```python
from build123d import *

# Parameters (mm, degrees)
BASE_SKETCH_W                   = 16
BASE_SKETCH_H                   = 20
BASE_EXTRUDE_DEPTH              = 12
TOP_START                       = 10
PROTRUSION_SKETCH_R             = 5
TOP_PROTRUSION_EXTRUDE_DEPTH    = 2
BOTTOM_START                    = -10
PROTRUSION_SKETCH_2_R           = 5
BOTTOM_PROTRUSION_EXTRUDE_DEPTH = 2
PROTRUSION_CHAMFER_SIZE         = 1
F_5_0MM_DOWEL_HOLE1_D           = 5
F_1_6MM_DOWEL_HOLE1_D           = 1.6
F_1_6MM_DOWEL_HOLE1_DEPTH       = 8
F_1_6MM_DOWEL_HOLE1_TIP         = 0.480688495
F_1_6_1_6_DIAMETER_HOLE4_D      = 1.6
F_1_6_1_6_DIAMETER_HOLE4_DEPTH  = 3.5
F_1_6_1_6_DIAMETER_HOLE4_TIP    = 0.480688495
M2X0_4_TAPPED_HOLE1_D           = 1.6
M2X0_4_TAPPED_HOLE1_DEPTH       = 4
M2X0_4_TAPPED_HOLE1_TIP         = 0.480688495
M2X0_4_TAPPED_HOLE2_D           = 1.6
M2X0_4_TAPPED_HOLE2_DEPTH       = 4
M2X0_4_TAPPED_HOLE2_TIP         = 0.480688495
F_2_2_2_2_DIAMETER_HOLE1_D      = 2.2
F_1_3_1_3_DIAMETER_HOLE1_D      = 1.3
F_1_3_1_3_DIAMETER_HOLE1_DEPTH  = 6
F_1_3_1_3_DIAMETER_HOLE1_TIP    = 0.390559402
F_1_3_1_3_DIAMETER_HOLE2_D      = 1.3
F_1_3_1_3_DIAMETER_HOLE2_DEPTH  = 6
F_1_3_1_3_DIAMETER_HOLE2_TIP    = 0.390559402
F_1_3_1_3_DIAMETER_HOLE3_D      = 1.3
F_1_3_1_3_DIAMETER_HOLE3_DEPTH  = 6
F_1_3_1_3_DIAMETER_HOLE3_TIP    = 0.390559402


with BuildPart() as part:
    # Base Sketch → Base Extrude (new body)
    with BuildSketch(Plane(origin=(0, 0, 0), x_dir=(1, 0, 0), z_dir=(0, 1, 0))):
        Rectangle(BASE_SKETCH_W, BASE_SKETCH_H)
    extrude(amount=BASE_EXTRUDE_DEPTH)

    # Protrusion Sketch → Top Protrusion Extrude (add)
    with BuildSketch(Plane.XY.offset(TOP_START)):
        with Locations((0, 6)):
            Circle(PROTRUSION_SKETCH_R)
    extrude(amount=TOP_PROTRUSION_EXTRUDE_DEPTH)

    # Protrusion Sketch<2> → Bottom Protrusion Extrude (add)
    with BuildSketch(Plane.XY.offset(BOTTOM_START)):
        with Locations((0, 6)):
            Circle(PROTRUSION_SKETCH_2_R)
    extrude(amount=-BOTTOM_PROTRUSION_EXTRUDE_DEPTH)

    # Protrusion Chamfer
    protrusion_chamfer_edges = [part.edges().sort_by_distance(p)[0] for p in [
        (-5, 6, 12),
        (-5, 6, -12),
    ]]
    chamfer(protrusion_chamfer_edges, length=PROTRUSION_CHAMFER_SIZE)

    # Ø5.0mm Dowel Hole1 (through all)
    with Locations(Plane.XY.offset(12)):
        with Locations((0, 6)):
            Hole(F_5_0MM_DOWEL_HOLE1_D / 2)

    # Ø1.6mm Dowel Hole1
    with Locations(Plane(origin=(8, 0, 0), x_dir=(0, 0, -1), z_dir=(1, 0, 0))):
        with Locations((0, 6)):
            Hole(F_1_6MM_DOWEL_HOLE1_D / 2, depth=F_1_6MM_DOWEL_HOLE1_DEPTH)
            with Locations((0, 0, -(F_1_6MM_DOWEL_HOLE1_DEPTH + F_1_6MM_DOWEL_HOLE1_TIP / 2))):  # 118° drill point
                Cone(0, F_1_6MM_DOWEL_HOLE1_D / 2, F_1_6MM_DOWEL_HOLE1_TIP, mode=Mode.SUBTRACT)

    # Ø1.6 (1.6) Diameter Hole4
    with Locations(Plane.ZY.offset(8)):
        with Locations((0, 6)):
            Hole(F_1_6_1_6_DIAMETER_HOLE4_D / 2, depth=F_1_6_1_6_DIAMETER_HOLE4_DEPTH)
            with Locations((0, 0, -(F_1_6_1_6_DIAMETER_HOLE4_DEPTH + F_1_6_1_6_DIAMETER_HOLE4_TIP / 2))):  # 118° drill point
                Cone(0, F_1_6_1_6_DIAMETER_HOLE4_D / 2, F_1_6_1_6_DIAMETER_HOLE4_TIP, mode=Mode.SUBTRACT)

    # M2x0.4 Tapped Hole1
    with Locations(Plane(origin=(8, 0, 0), x_dir=(0, 0, -1), z_dir=(1, 0, 0))):
        with Locations((-4.5, 6), (4.5, 6)):
            Hole(M2X0_4_TAPPED_HOLE1_D / 2, depth=M2X0_4_TAPPED_HOLE1_DEPTH)
            with Locations((0, 0, -(M2X0_4_TAPPED_HOLE1_DEPTH + M2X0_4_TAPPED_HOLE1_TIP / 2))):  # 118° drill point
                Cone(0, M2X0_4_TAPPED_HOLE1_D / 2, M2X0_4_TAPPED_HOLE1_TIP, mode=Mode.SUBTRACT)

    # M2x0.4 Tapped Hole2
    with Locations(Plane.ZY.offset(8)):
        with Locations((-4.5, 6), (4.5, 6)):
            Hole(M2X0_4_TAPPED_HOLE2_D / 2, depth=M2X0_4_TAPPED_HOLE2_DEPTH)
            with Locations((0, 0, -(M2X0_4_TAPPED_HOLE2_DEPTH + M2X0_4_TAPPED_HOLE2_TIP / 2))):  # 118° drill point
                Cone(0, M2X0_4_TAPPED_HOLE2_D / 2, M2X0_4_TAPPED_HOLE2_TIP, mode=Mode.SUBTRACT)

    # Ø2.2 (2.2) Diameter Hole1 (through all)
    with Locations(Plane(origin=(0, 12, 0), x_dir=(1, 0, 0), z_dir=(0, 1, 0))):
        with Locations((-5, 7), (5, 7), (-5, -7), (5, -7)):
            Hole(F_2_2_2_2_DIAMETER_HOLE1_D / 2)

    # Ø1.3 (1.3) Diameter Hole1
    with Locations(Plane(origin=(0, 0, 0), x_dir=(-1, 0, 0), z_dir=(0, -1, 0))):
        with Locations((0, 7.5), (0, -7.5)):
            Hole(F_1_3_1_3_DIAMETER_HOLE1_D / 2, depth=F_1_3_1_3_DIAMETER_HOLE1_DEPTH)
            with Locations((0, 0, -(F_1_3_1_3_DIAMETER_HOLE1_DEPTH + F_1_3_1_3_DIAMETER_HOLE1_TIP / 2))):  # 118° drill point
                Cone(0, F_1_3_1_3_DIAMETER_HOLE1_D / 2, F_1_3_1_3_DIAMETER_HOLE1_TIP, mode=Mode.SUBTRACT)

    # Ø1.3 (1.3) Diameter Hole2
    with Locations(Plane(origin=(0, 0, 0), x_dir=(-1, 0, 0), z_dir=(0, -1, 0))):
        with Locations((5, 0)):
            Hole(F_1_3_1_3_DIAMETER_HOLE2_D / 2, depth=F_1_3_1_3_DIAMETER_HOLE2_DEPTH)
            with Locations((0, 0, -(F_1_3_1_3_DIAMETER_HOLE2_DEPTH + F_1_3_1_3_DIAMETER_HOLE2_TIP / 2))):  # 118° drill point
                Cone(0, F_1_3_1_3_DIAMETER_HOLE2_D / 2, F_1_3_1_3_DIAMETER_HOLE2_TIP, mode=Mode.SUBTRACT)

    # Ø1.3 (1.3) Diameter Hole3
    with Locations(Plane(origin=(0, 12, 0), x_dir=(1, 0, 0), z_dir=(0, 1, 0))):
        with Locations((0, -7.5), (0, -3), (0, 3), (0, 7.5)):
            Hole(F_1_3_1_3_DIAMETER_HOLE3_D / 2, depth=F_1_3_1_3_DIAMETER_HOLE3_DEPTH)
            with Locations((0, 0, -(F_1_3_1_3_DIAMETER_HOLE3_DEPTH + F_1_3_1_3_DIAMETER_HOLE3_TIP / 2))):  # 118° drill point
                Cone(0, F_1_3_1_3_DIAMETER_HOLE3_D / 2, F_1_3_1_3_DIAMETER_HOLE3_TIP, mode=Mode.SUBTRACT)


solid = part.part
```
Part model, mm, in its own coordinate system. A direction names the side the tool comes from. Round coordinates to 2 decimals unless told otherwise and drop trailing zeros. Order: outer loops, then holes, each group sorted by start corner. A loop starts at its lowest first (then second) coordinate and runs counter-clockwise, first axis right, second up. Notation, with made-up numbers: M 18.25,-30 L 23.25,-30 A28 ccw 23.25,-6 Z; hole C 41.5,65 d5. An arc over 180 degrees is marked long. Answer in a Markdown table with one row per item. Add a question column.
Q1. Cut at C-C on z = 9.25. Give the cut face in (x, y).
Q2. Wall check: L1, parallel to Z at x = 0, y = 2.25; L2, parallel to Z at x = 5, y = 2.75; L3, parallel to Z at x = 0, y = 9.3. Give the ranges that are in metal, low to high. Write a range as from..to.
Q3. Pin check, flat tips, straight feed: pin 1 (1 mm diameter, centred on x = 0, z = -3, fed in from +Y); pin 2 (1 mm diameter, centred on x = 0, z = -7.5, fed in from +Y); pin 3 (2.5 mm diameter, centred on y = 6, z = -4.5, fed in from +X); pin 4 (1.3 mm diameter, centred on y = 6, z = 4.5, fed in from +X). Stop position of each tip, or through.
Q4. Cut at A-A on x = 6.5. Give the cut face in (y, z).
Q5. Cut at D-D on x = 0. Give the number of separate pieces and of enclosed holes in the cut face, and give its area (3 significant figures).
Q6. 3-axis set-ups, long thin cutter, end or side, ignore diameter. For faces 4 (the face through (-5.97, 6.54, -3.91)), 5 (the face through (-1.08, 1.12, 10.49)), 6 (the face through (-4.38, 2.81, -0.2)), 7 (the face through (5.97, 6.54, -5.09)): which of +Z, -Z, +X, -X, +Y, -Y reach the whole face in a straight line?
Q7. Mould opens along X. For faces 1 (the face through (-5.4, 5.9, 10)), 2 (the face through (-4.103, 6.138, -0.018)), 3 (the face through (0.35, 1.82, -8.05)) say: +X half, -X half, draft (parallel to the pull), parting line (faces both ways), or undercut.
Q8. Cut at B-B on z = -3. Give the cut face in (x, y).
Established:
| question | item | result |
|---|---|---|
| 1 | outline | M -8,0 L 8,0 L 8,12 L -8,12 Z; hole C 0,6 d5 |
| 2 | L1 | z = -12..-8.15, -6.85..6.85, 8.15..12 |
| 2 | L2 | z = -10..-8.1, -5.9..5.9, 8.1..10 |
| 2 | L3 | z = -12..-8.15, -6.85..-3.65, -2.35..2.35, 3.65..6.85, 8.15..12 |
| 3 | pin 1 | stops at y = 3.55 |
| 3 | pin 2 | passes through |
| 3 | pin 3 | stops at x = 8 |
| 3 | pin 4 | stops at x = 3.91 |
| 4 | outline | M 0,-10 L 12,-10 L 12,10 L 0,10 Z; hole C 6,-4.5 d1.6; hole C 6,0 d1.6; hole C 6,4.5 d1.6 |
| 5 | separate pieces | 8 |
| 5 | enclosed holes | 0 |
| 5 | area | 131 mm2 |
| 6 | face 4 | -X |
| 6 | face 5 | +Z |
| 6 | face 6 | -Y |
| 6 | face 7 | +X |
| 7 | face 1 | draft |
| 7 | face 2 | -X half |
| 7 | face 3 | undercut |
| 8 | outline | M -8,0 L 8,0 L 8,12 L 0.65,12 L 0.65,8.41 A2.5 cw long -0.65,8.41 L -0.65,12 L -8,12 Z |
